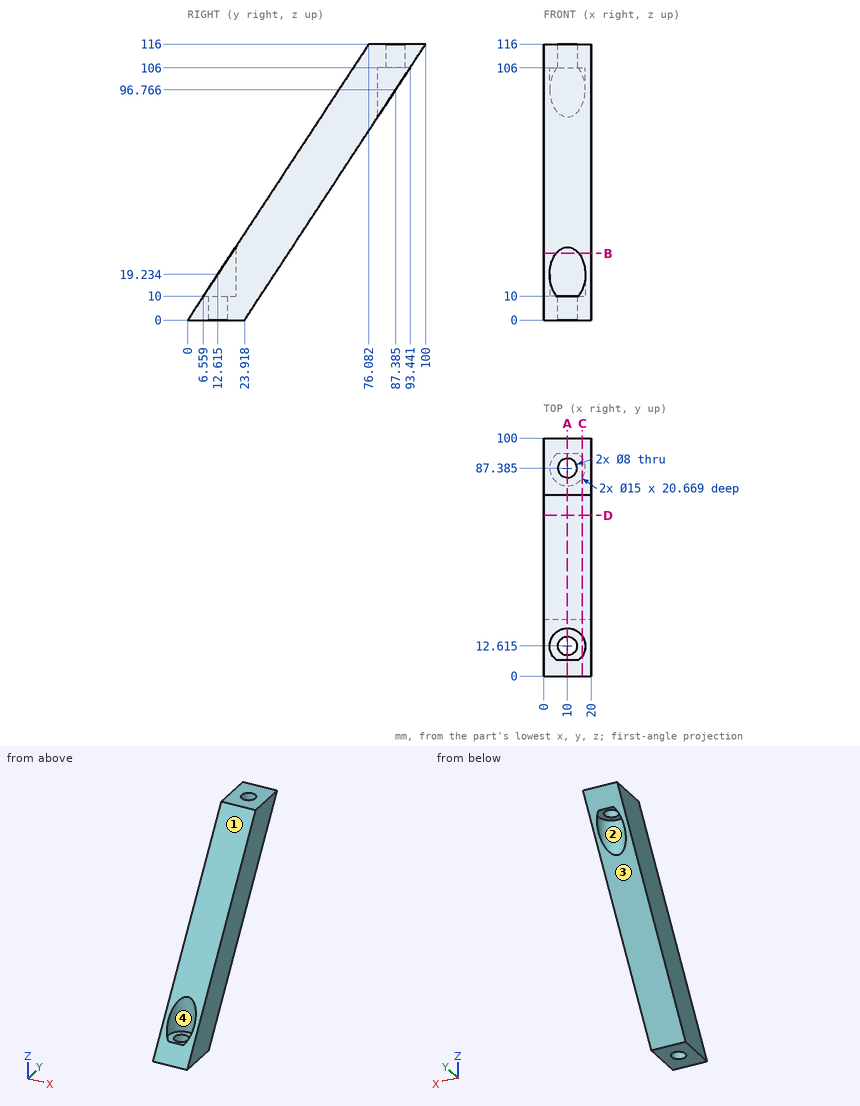
Input: dimensioned drawing with shaded views. Units: mm. Origin: part minimum x, y, z. A direction names the side the tool comes from. Coordinates: 2 decimals unless noted, no trailing zeros. Write each loop counter-clockwise with the first axis right and the second up, starting at its lowest first coordinate (ties: lowest second). Pieces come first, ordered by that corner, then holes. Notation, with made-up numbers: (-6, 13.5) -> (47, 13.5) arc R20 cw to (47, 38.5) -> close; hole circle Ø10 at (-15.5, 0.5). An arc over 180 degrees is marked (long way). Return JSON: item names as keys, results as strings. Group by question number.
1) Section query A-A, the plane x = 10. Return loops of the section in (y, z) (1 decimal).
2) Section query C-C, the plane x = 16.25. Return loops of the section in (y, z) (1 decimal), plus the area to 3 significant figures.
3) Mould query, pull axis X, two halves, no side actions, for the marked faces 1 and 2. Classes: +X half, -X half, draft (parallel to the pull), parting line (faces both ways), or undercut.
4) Section query D-D, the plane y = 67.5. Return loops of the section in (x, z) (1 decimal).
5) Set-up query: the marked faces 3 and 4. Return all of +Z, -Z, +X, -X, +Y, -Y with unobstructed straight access to the full face (end or side cutting, diameter ignored); none if empty.
6) Contact query for flat-ended pins moving along their axis: P1, Ø7, axis at x = 10, y = 87.39, coming from the +Z side; P2, Ø8, axis at x = 16, y = 84.5, coming from the -Z side; P3, Ø1.5, axis at x = 14, z = 30.5, coming from the +Y side (1 decimal); P4, Ø1, axis at x = 2.5, z = 25.5, coming from the +Y side. Output: stop coordinate, or through.
7) Ray query, line 1 along Z through (x, y) = (10.25, 19); line 2 along Z through (x, y) = (9.5, 61) (1 decimal); line 3 along Y through (x, z) = (10, 5.25) (1 decimal). Return the intervals inside material, ascending.
8) Section query B-B, the plane z = 28. Return loops of the section in (x, y) (1 decimal).
From the geometry:
{
 "1": {"outline": "(0, 0) -> (8.6, 0) -> (8.6, 10) -> (6.6, 10) -> close; (16.6, 0) -> (23.9, 0) -> (79.9, 85.3) -> (79.9, 106) -> (83.4, 106) -> (83.4, 116) -> (76.1, 116) -> (20.1, 30.7) -> (20.1, 10) -> (16.6, 10) -> close; (91.4, 106) -> (93.4, 106) -> (100, 116) -> (91.4, 116) -> close"},
 "2": {"outline": "(0, 0) -> (23.9, 0) -> (83.2, 90.4) -> (83.2, 106) -> (91.5, 106) -> (91.5, 103.1) -> (100, 116) -> (76.1, 116) -> (16.8, 25.6) -> (16.8, 10) -> (8.5, 10) -> (8.5, 12.9) -> close", "area": "2,620 mm²"},
 "3": {"face 1": "draft", "face 2": "undercut"},
 "4": {"outline": "(0, 66.4) -> (20, 66.4) -> (20, 102.9) -> (0, 102.9) -> close"},
 "5": {"face 3": "-Z, +X, -X, +Y", "face 4": "+Z"},
 "6": {"P1": "through", "P2": "z = 86.27", "P3": "y = 44.4", "P4": "y = 40.97"},
 "7": {"line 1": "0 to 10", "line 2": "56.5 to 93", "line 3": "3.4 to 8.6, 16.6 to 27.4"},
 "8": {"outline": "(0, 18.4) -> (5.2, 18.4) arc R7.5 cw to (14.8, 18.4) -> (20, 18.4) -> (20, 42.3) -> (0, 42.3) -> close"}
}
